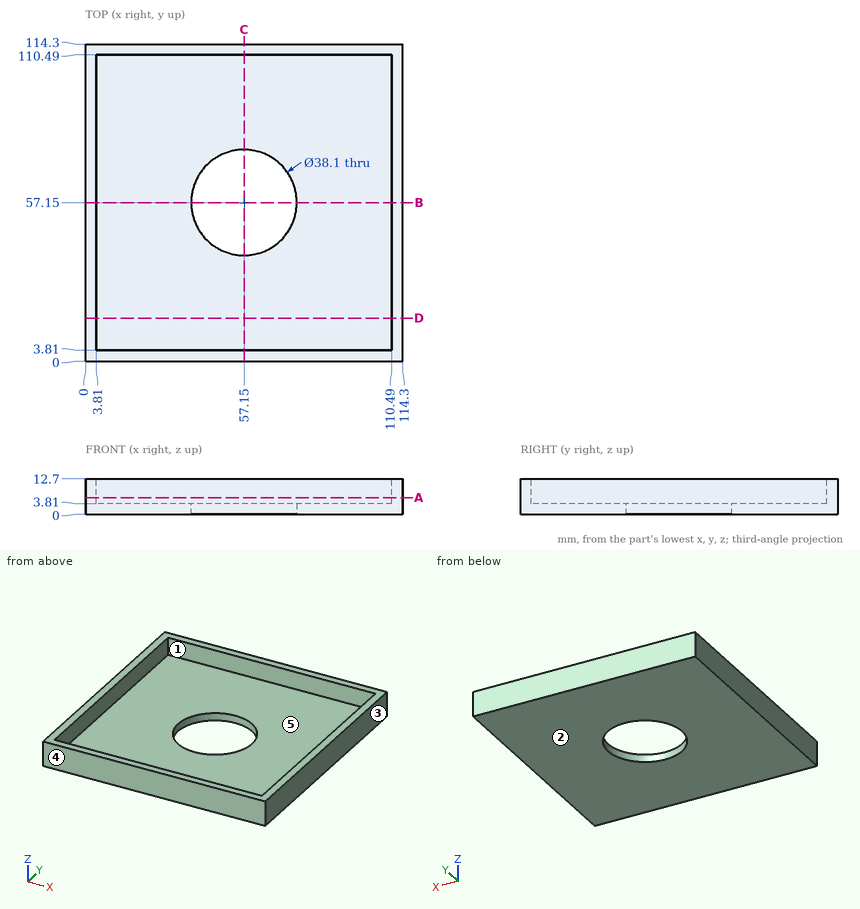
Geometry check sheet. Reference: drawing and pictorial views, mm from the part's lowest x, y, z. A direction names the side the tool comes from. Give positions to 0.01 mm unless a question says otherwise; leave off trailing zeros. Order: outer loops, then holes, each group sorted by start corner. A loop starts at its lowest first (then second) coordinate and runs counter-clockwise, first axis right, second up. Notation, with made-up numbers: (-11.75, 33) -> (46.25, 33) arc R34 cw to (46.25, 69) -> close; hole circle Ø7 at (18, 60). An arc over 180 degrees is marked (long way). Write each question's results on one line, items separated by ' | '. Start each with the question number.
(1) Mould release check, pull along X, two halves, no side actions. Record for the marked faces 1, 2 and 3: pulls with the +X half, pulls with the -X half, needs draft (parallel to the pull), parting line crosses it, or undercut.
(2) Sectioned sample at D-D (y = 15.5). Enter the section's corners in (x, z).
(3) Access from +Z, -Z, +X, -X, +Y, -Y to the whole of each face (thin tool, end or side, straight path). Record for the marked faces 4 and 5.
(4) Sectioned sample at A-A (z = 6). Enter the section's corners in (x, y).
(5) Scan lines: line 1 (X direction, y = 22.5, z = 8.75); line 2 (Y direction, x = 57.15, z = 1.05). Record each from-to range of solid material in increasing order.
(6) Sectioned sample at B-B (y = 57.15). Enter the section's corners in (x, z).
(7) Gauge pin test, flat end, axial feed: P1, Ø12, axis at x = 98.5, y = 94.5, coming from the +Z side. Record the tip position at first contact, or that the pin passes through.
Answer below:
1) face 1: undercut | face 2: needs draft | face 3: pulls with the +X half
2) outline: (0, 0) -> (114.3, 0) -> (114.3, 12.7) -> (110.49, 12.7) -> (110.49, 3.81) -> (3.81, 3.81) -> (3.81, 12.7) -> (0, 12.7) -> close
3) face 4: +Z, -Z, +X, -X, -Y | face 5: +Z
4) outline: (0, 0) -> (114.3, 0) -> (114.3, 114.3) -> (0, 114.3) -> close; hole (3.81, 3.81) -> (110.49, 3.81) -> (110.49, 110.49) -> (3.81, 110.49) -> close
5) line 1: 0 to 3.81, 110.49 to 114.3 | line 2: 0 to 38.1, 76.2 to 114.3
6) outline: (0, 0) -> (38.1, 0) -> (38.1, 3.81) -> (3.81, 3.81) -> (3.81, 12.7) -> (0, 12.7) -> close; (76.2, 0) -> (114.3, 0) -> (114.3, 12.7) -> (110.49, 12.7) -> (110.49, 3.81) -> (76.2, 3.81) -> close
7) P1: z = 3.81
